from build123d import *

# Parameters (mm, degrees)
SKETCH1_R           = 2.2098
BOSS_EXTRUDE1_DEPTH = 6.20300004
SKETCH2_R           = 4.2164
CUT_EXTRUDE1_DEPTH  = 3.048
SKETCH3_R           = 2.2098
CUT_EXTRUDE2_DEPTH  = 66.670862713
SKETCH4_R           = 3.30699999
CUT_EXTRUDE3_DEPTH  = 1.906999996


with BuildPart() as part:
    # Sketch1 → Boss-Extrude1 (new body)
    with BuildSketch(Plane.XY):
        with BuildLine():
            Line((-50.8, -31.75), (50.8, -31.75))
            ThreePointArc((50.8, -31.75), (55.290128061, -29.890128061), (57.15, -25.4))
            Line((57.15, -25.4), (57.15, 25.4))
            ThreePointArc((57.15, 25.4), (55.290128061, 29.890128061), (50.8, 31.75))
            Line((50.8, 31.75), (-50.8, 31.75))
            ThreePointArc((-50.8, 31.75), (-55.290128061, 29.890128061), (-57.15, 25.4))
            Line((-57.15, 25.4), (-57.15, -25.4))
            ThreePointArc((-57.15, -25.4), (-55.290128061, -29.890128061), (-50.8, -31.75))
        make_face()
        with Locations((-50.8, -25.4)):
            Circle(SKETCH1_R, mode=Mode.SUBTRACT)
        with Locations((-50.8, 25.4)):
            Circle(SKETCH1_R, mode=Mode.SUBTRACT)
        with Locations((50.8, 25.4)):
            Circle(SKETCH1_R, mode=Mode.SUBTRACT)
        with Locations((50.8, -25.4)):
            Circle(SKETCH1_R, mode=Mode.SUBTRACT)
    extrude(amount=BOSS_EXTRUDE1_DEPTH)

    # Sketch2 → Cut-Extrude1 (cut)
    with BuildSketch(Plane.XY.offset(6.20300004)):
        with Locations((-50.8, 25.4)):
            Circle(SKETCH2_R)
        with Locations((50.8, 25.4)):
            Circle(SKETCH2_R)
        with Locations((50.8, -25.4)):
            Circle(SKETCH2_R)
        with Locations((-50.8, -25.4)):
            Circle(SKETCH2_R)
    extrude(amount=-CUT_EXTRUDE1_DEPTH, mode=Mode.SUBTRACT)

    # Sketch3 → Cut-Extrude2 (cut, through all)
    with BuildSketch(Plane.XY.offset(6.20300004)):
        with Locations((-38.1, 25.4)):
            Circle(SKETCH3_R)
        with Locations(Location((38.1, 25.4, 0), (0, 0, 180))):
            Circle(SKETCH3_R)
        with Locations((38.1, -25.4)):
            Circle(SKETCH3_R)
        with Locations(Location((-38.1, -25.4, 0), (0, 0, 180))):
            Circle(SKETCH3_R)
    extrude(amount=-CUT_EXTRUDE2_DEPTH, mode=Mode.SUBTRACT)

    # Sketch4 → Cut-Extrude3 (cut)
    with BuildSketch(Plane.XY.offset(6.20300004)):
        with Locations((-38.1, 25.4)):
            Circle(SKETCH4_R)
        with Locations((38.1, 25.4)):
            Circle(SKETCH4_R)
        with Locations((38.1, -25.4)):
            Circle(SKETCH4_R)
        with Locations((-38.1, -25.4)):
            Circle(SKETCH4_R)
    extrude(amount=-CUT_EXTRUDE3_DEPTH, mode=Mode.SUBTRACT)


solid = part.part
CAD build for the part. Positions are in the model's coordinates, mm. A direction names the side the tool comes from. Give positions to 0.01 mm unless a question says otherwise; leave off trailing zeros. Order: outer loops, then holes, each group sorted by start corner. A loop starts at its lowest first (then second) coordinate and runs counter-clockwise, first axis right, second up. Notation, with made-up numbers: (68, -19) -> (124, -19) arc R10 cw to (124, -15) -> close; hole circle Ø11 at (89, 64). An arc over 180 degrees is marked (long way). Return JSON: item names as keys, results as strings.
Q1. Saw through at B-B (z = 2). Count the separate pieces of the cut face and the enclosed holes in it, then the cut area to 3 significant figures.
Working result:
{"separate pieces": "1", "enclosed holes": "8", "area": "7,100 mm²"}
Q2. Which spindle directions (+Z, -Z, +X, -X, +Y, -Y) get a long thin tool onto all of the face, cutting with end or side? Do faces 1 (the face through (55.34, 29.84, 3.06)), 2 (the face through (-34.946, 26.393, 5.263)). Say none if no direction does.
Working result:
{"face 1": "+Z, -Z, +X, +Y", "face 2": "+Z"}
Q3. Mould opens along X. For faces 3 (the face through (52.91, 26.06, 1.56)), 4 (the face through (57.15, 0, 3)), 5 (the face through (-55.34, -29.84, 3.06)), 6 (the face through (39, 23, 4.296)) say: pulls with the +X half, pulls with the -X half, needs draft (parallel to the pull), parting line crosses it, or undercut.
Working result:
{"face 3": "undercut", "face 4": "pulls with the +X half", "face 5": "pulls with the -X half", "face 6": "undercut"}
Q4. Flat gauge pins, fed straight in: pin 1 (3.5 mm diameter, centred on x = -38.1, y = -25.4, fed in from +Z); pin 2 (7 mm diameter, centred on x = 50.8, y = -25.4, fed in from +Z) (3 decimals). Where does each tip first touch, or does it go through?
Working result:
{"pin 1": "through", "pin 2": "z = 3.155"}
Q5. Saw through at A-A (x = -38.1). Write the cut outline in (y, z), then the cut area to 3 significant figures.
Working result:
{"outline": "(-31.75, 0) -> (-27.61, 0) -> (-27.61, 4.3) -> (-28.71, 4.3) -> (-28.71, 6.2) -> (-31.75, 6.2) -> close; (-23.19, 0) -> (23.19, 0) -> (23.19, 4.3) -> (22.09, 4.3) -> (22.09, 6.2) -> (-22.09, 6.2) -> (-22.09, 4.3) -> (-23.19, 4.3) -> close; (27.61, 0) -> (31.75, 0) -> (31.75, 6.2) -> (28.71, 6.2) -> (28.71, 4.3) -> (27.61, 4.3) -> close", "area": "331 mm²"}
Q6. Drill centre lines: line 1 (Y direction, x = 38.1, z = 5.5); line 2 (Y direction, x = 50.8, z = 4.8); line 3 (X direction, y = -25.5, z = 2). Where is each one in solid material? Low to high.
Working result:
{"line 1": "-31.75 to -28.71, -22.09 to 22.09, 28.71 to 31.75", "line 2": "-31.75 to -29.62, -21.18 to 21.18, 29.62 to 31.75", "line 3": "-57.15 to -53.01, -48.59 to -40.31, -35.89 to 35.89, 40.31 to 48.59, 53.01 to 57.15"}
